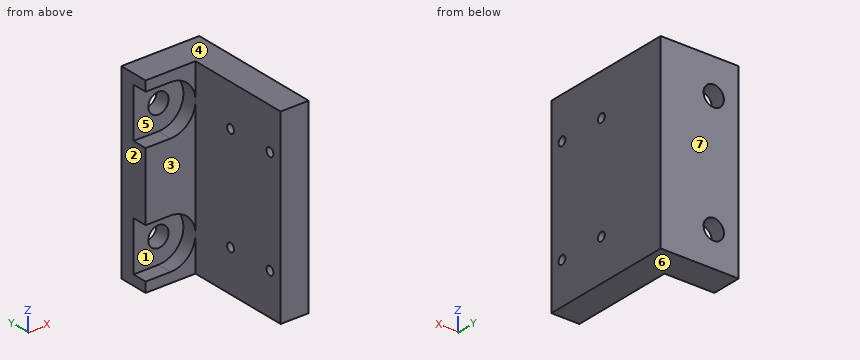
from build123d import *

# Parameters (mm, degrees)
MAINBODY_EXTRUDE_START                    = 293.6
MAINBODY_EXTRUDE_DEPTH                    = 39.8
BOLSTEREDPLINTH_EXTRUDE_START             = -3.4
BOLSTEREDPLINTH_EXTRUDE_DEPTH             = 39.8
PROXIMALMOUNTHOLESCREWHEADLANDS_CUT_START = -6.35
PROXIMALMOUNTHOLESCREWHEADLANDS_CUT_DEPTH = 3.175
PROXIMALMOUNTSCREWHOLES_SKETCH_R          = 2.15
PROXIMALMOUNTHOLES_CUT_DEPTH              = 335.794235324
LIMITSWITCHMOUNTHOLES_HOLEWIZARD_D        = 1.8


with BuildPart() as part:
    # projectionZ_sketch → mainBody_extrude (new body)
    with BuildSketch(Plane.XY.offset(MAINBODY_EXTRUDE_START)):
        Polygon((3.175, -28.6375), (0, -28.6375), (0, -3.175), (-10.56, -3.175), (-10.56, 0), (3.175, 0), align=None)
    extrude(amount=MAINBODY_EXTRUDE_DEPTH)

    # bolsteredPlinthProjectionZ_sketch → bolsteredPlinth_extrude (add)
    with BuildSketch(Plane.XY.offset(297).offset(BOLSTEREDPLINTH_EXTRUDE_START)):
        Polygon((-10.56, 0), (5.935, 0), (5.935, -28.6375), (3.175, -28.6375), (0, -6.35), (-10.56, -6.35), align=None)
    extrude(amount=BOLSTEREDPLINTH_EXTRUDE_DEPTH)

    # proximalMountScrewHeadLands_sketch → proximalMountHoleScrewHeadLands_cut (cut)
    with BuildSketch(Plane(origin=(0, 0, 0), x_dir=(1, 0, 0), z_dir=(0, 1, 0)).offset(PROXIMALMOUNTHOLESCREWHEADLANDS_CUT_START)):
        with BuildLine():
            Line((-10.56, -331.280000019), (-5.28, -331.280000019))
            ThreePointArc((-5.28, -331.280000019), (0, -326.000000019), (-5.28, -320.720000019))
            Line((-5.28, -320.720000019), (-10.56, -320.720000019))
            Line((-10.56, -320.720000019), (-10.56, -331.280000019))
        make_face()
        with BuildLine():
            Line((-10.56, -306.279999981), (-5.28, -306.279999981))
            ThreePointArc((-5.28, -306.279999981), (0, -300.999999981), (-5.28, -295.719999981))
            Line((-5.28, -295.719999981), (-10.56, -295.719999981))
            Line((-10.56, -295.719999981), (-10.56, -306.279999981))
        make_face()
    extrude(amount=PROXIMALMOUNTHOLESCREWHEADLANDS_CUT_DEPTH, mode=Mode.SUBTRACT)

    # proximalMountScrewHoles_sketch → proximalMountHoles_cut (cut, through all)
    with BuildSketch(Plane(origin=(0, 0, 0), x_dir=(1, 0, 0), z_dir=(0, 1, 0))):
        with Locations(Location((-5.28, -326.000000019, 0), (0, 0, 270))):
            Circle(PROXIMALMOUNTSCREWHOLES_SKETCH_R)
        with Locations(Location((-5.28, -300.999999981, 0), (0, 0, 270))):
            Circle(PROXIMALMOUNTSCREWHOLES_SKETCH_R)
    extrude(amount=-PROXIMALMOUNTHOLES_CUT_DEPTH, mode=Mode.SUBTRACT)

    # limitSwitchMountHoles_holeWizard (through all)
    with Locations(Plane(origin=(0, 0, 0), x_dir=(0, 0, -1), z_dir=(-1, 0, 0))):
        with Locations((-302.4, 25.8375), (-302.4, 15.5375), (-324.6, 15.5375), (-324.6, 25.8375)):
            Hole(LIMITSWITCHMOUNTHOLES_HOLEWIZARD_D / 2)


solid = part.part
Read the model definition and answer for the solid it produces. Units are mm, in the model's axes. Face numbers are marked on the shaded views. A direction names the side the tool comes from. Give positions to 0.01 mm unless a question says otherwise; leave off trailing zeros. Write each loop counter-clockwise with the first axis right and the second up, starting at its lowest first coordinate (ties: lowest second). Pieces come first, ordered by that corner, then holes. Notation, with made-up numbers: (-12.75, 2) - (37.25, 2) arc R27 cw to (37.25, 31) - close; hole circle Ø6 at (73.25, 24.25). An arc over 180 degrees is marked (long way). Return JSON: item names as keys, results as strings.
Q1. A cutting plane is placed at A-A, the plane z = 302.4. Count the separate pieces of the cut face and the enclosed holes in it, and give its area (3 significant figures).
Reply:
{"separate pieces": "4", "enclosed holes": "0", "area": "172 mm²"}
Q2. Given P1, Ø2.5, axis at y = -15.54, z = 324.6, coming from the +X side (3 decimals); P2, Ø3.5, axis at x = -7, z = 329, coming from the -Y side (3 decimals); P3, Ø1, axis at y = -8.5, z = 316.5, coming from the -X side; P4, Ø3, axis at x = -4, z = 321.5, coming from the -Y side, each flat-ended and moving along its own axis, determine where each tip first touches the part or whether it passes through.
Reply:
{"P1": "x = 5.935", "P2": "y = -3.175", "P3": "x = 0", "P4": "y = -6.35"}
Q3. A cutting plane is placed at B-B, the plane x = -1. Determine the outline of the cut face in (y, z) (3 decimals).
Reply:
{"outline": "(-6.35, 293.6) - (0, 293.6) - (0, 333.4) - (-6.35, 333.4) - (-6.35, 329.092) - (-3.175, 329.092) - (-3.175, 322.908) - (-6.35, 322.908) - (-6.35, 304.092) - (-3.175, 304.092) - (-3.175, 297.908) - (-6.35, 297.908) - close"}
Q4. Consider line 1 along Y through (x, z) = (3.95, 324.6); line 2 along X through (y, z) = (-1.1, 301) (3 decimals); line 3 along Z through (x, y) = (2.25, -25.5). Determine where each line is inside the solid, lowest interval first. Write a range as [from, to].
Reply:
{"line 1": "[-28.64, -26.74], [-24.94, -16.44], [-14.64, 0]", "line 2": "[-10.56, -7.43], [-3.13, 5.935]", "line 3": "[293.6, 301.57], [303.23, 323.77], [325.43, 333.4]"}
Q5. A cutting plane is placed at D-D, the plane y = -20. Determine the outline of the cut face in (x, z) (3 decimals).
Reply:
{"outline": "(0, 293.6) - (5.935, 293.6) - (5.935, 333.4) - (0, 333.4) - close"}
Q6. For a pull along Z with two mould halves and no side action, classify the marked faces 4, 5, 6 and 7 as released by +Z, released by -Z, zero draft, split by the parting line, or undercut.
Reply:
{"face 4": "released by +Z", "face 5": "undercut", "face 6": "released by -Z", "face 7": "zero draft"}
Q7. For the marked faces 1, 2 and 3, determine the directions among +Z, -Z, +X, -X, +Y, -Y from which every point of the face is accessible in a straight line to the end or side of a thin tool.
Reply:
{"face 1": "-X, -Y", "face 2": "+Z, -Z, -X, +Y, -Y", "face 3": "+Z, -Z, -X, -Y"}
